```python
from build123d import *

# Parameters (mm, degrees)
SKETCH1_W           = 76.2
SKETCH1_H           = 76.2
SKETCH1_W_2         = 68.58
SKETCH1_H_2         = 68.58
BOSS_EXTRUDE1_DEPTH = 457.2
SKETCH2_R           = 13.335
CUT_EXTRUDE1_DEPTH  = 914.4
SKETCH3_R           = 5.08
CUT_EXTRUDE2_DEPTH  = 914.4


with BuildPart() as part:
    # Sketch1 → Boss-Extrude1 (new body)
    with BuildSketch(Plane(origin=(0, 0, 0), x_dir=(1, 0, 0), z_dir=(0, 1, 0))):
        with Locations((38.1, 38.1)):
            Rectangle(SKETCH1_W, SKETCH1_H)
        with Locations((38.1, 38.1)):
            Rectangle(SKETCH1_W_2, SKETCH1_H_2, mode=Mode.SUBTRACT)
    extrude(amount=BOSS_EXTRUDE1_DEPTH)

    # Sketch2 → Cut-Extrude1 (cut)
    with BuildSketch(Plane.ZY):
        with Locations((-38.1, 228.6)):
            Circle(SKETCH2_R)
    extrude(amount=-CUT_EXTRUDE1_DEPTH, mode=Mode.SUBTRACT)

    # Sketch3 → Cut-Extrude2 (cut)
    with BuildSketch(Plane.ZY):
        with Locations((-57.742411839, 248.242411839)):
            Circle(SKETCH3_R)
        with Locations((-18.457588161, 248.242411839)):
            Circle(SKETCH3_R)
        with Locations((-57.742411839, 208.957588161)):
            Circle(SKETCH3_R)
        with Locations((-18.457588161, 208.957588161)):
            Circle(SKETCH3_R)
    extrude(amount=-CUT_EXTRUDE2_DEPTH, mode=Mode.SUBTRACT)


solid = part.part
```
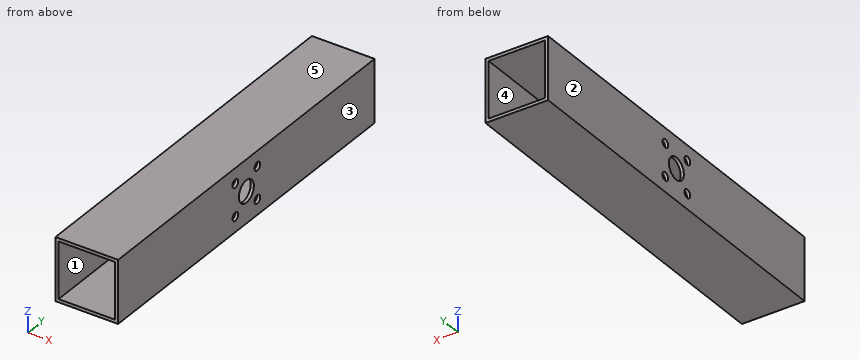
Can you work these out from the model? Positions are in its coordinate system, mm. Face numbers are marked on the shaded views. A direction names the side the tool comes from. Give positions to 0.01 mm unless a question says otherwise; leave off trailing zeros. Loops run counter-clockwise (first coordinate to the right, second up) from the corner with the lowest first, then second, coordinate; pieces in that order, holes last. Notation, with made-up numbers: M 22.25,15 L 52.25,15 A21 ccw 52.25,45 Z; hole C 52.25,76 d1. An arc over 180 degrees is marked long. One line per question, with ' | ' between items. Start each with the question number.
Q1. If we section it at B-B (y = 228.6): Please give me the cut outline in (x, z) (3 decimals).
Q2. If we mould it in two halves opening along X, with no side actions, what happens to the marked faces 1, 2 and 3? For each: +X half, -X half, draft (parallel to the pull), parting line (faces both ways), or undercut.
Q3. If I drill on line 1 (Z direction, x = 49.5, y = 112); line 2 (X direction, y = 263.5, z = -71.5), over which ranges is the centre line in solid material (lowest first)? Write a range as from..to.
Q4. If we section it at A-A (z = -38.1): Please give me the cut outline in (x, y) (3 decimals), plus the area to 3 significant figures.
Q5. If we section it at C-C (x = 55.5): Please give me the cut outline in (y, z), plus the area to 3 significant figures.
Q6. For the marked faces 4 and 5, which set-ups out of +Z, -Z, +X, -X, +Y, -Y let a thin tool reach every point of the face, with its end or its side?
Q7. If we section it at D-D (y = 146.5): Please give me the cut outline in (x, z), plus the area to 3 significant figures.
Q8. For pin 1 Ø11.5 at (y, z) = (208.96, -18.46) entering from +X, with a flat end and sliding along its axis, tell me the tip position at first contact or that it passes through.
Computed:
1) outline: M 0,-76.2 L 76.2,-76.2 L 76.2,-51.435 L 72.39,-51.435 L 72.39,-72.39 L 3.81,-72.39 L 3.81,-51.435 L 0,-51.435 Z; M 0,-24.765 L 3.81,-24.765 L 3.81,-3.81 L 72.39,-3.81 L 72.39,-24.765 L 76.2,-24.765 L 76.2,0 L 0,0 Z
2) face 1: undercut | face 2: -X half | face 3: +X half
3) line 1: z = -76.2..-72.39, -3.81..0 | line 2: x = 0..3.81, 72.39..76.2
4) outline: M 0,0 L 3.81,0 L 3.81,215.265 L 0,215.265 Z; M 0,241.935 L 3.81,241.935 L 3.81,457.2 L 0,457.2 Z; M 72.39,0 L 76.2,0 L 76.2,215.265 L 72.39,215.265 Z; M 72.39,241.935 L 76.2,241.935 L 76.2,457.2 L 72.39,457.2 Z | area: 3,280 mm²
5) outline: M 0,-76.2 L 457.2,-76.2 L 457.2,-72.39 L 0,-72.39 Z; M 0,-3.81 L 457.2,-3.81 L 457.2,0 L 0,0 Z | area: 3,480 mm²
6) face 4: +Y, -Y | face 5: +Z, +X, -X, +Y, -Y
7) outline: M 0,-76.2 L 76.2,-76.2 L 76.2,0 L 0,0 Z; hole M 3.81,-72.39 L 72.39,-72.39 L 72.39,-3.81 L 3.81,-3.81 Z | area: 1,100 mm²
8) pin 1: stops at x = 76.2
